Build history of the part. All positions in model axes, mm. Round coordinates to 2 decimals unless told otherwise and drop trailing zeros. Loops run counter-clockwise (first coordinate to the right, second up) from the corner with the lowest first, then second, coordinate; pieces in that order, holes last. Notation, with made-up numbers: (67, -7) -> (94, -7) arc R10 ccw to (94, 11) -> close; hole circle Ø9 at (-5.75, 30). An arc over 180 degrees is marked (long way). Put each result on its own line as item: value. Start each with the question number.
Item 1: Drill centre lines: probe 1 along X at (y, z) = (64, 114); probe 2 along Y at (x, z) = (22.5, 61.5); probe 3 along X at (y, z) = (94, 33.5). Where is each one in solid material? Low to high. Write a range as [from, to].
Item 2: Cut at B-B, the plane x = 59. List the corners of the cut face in (y, z), plus the area to 3 significant figures.
Item 3: Cut at A-A, the plane y = 12.5. List the corners of the cut face in (x, z).
Item 4: Cut at C-C, the plane z = 74.5. List the corners of the cut face in (x, y), plus the area to 3 significant figures.
Item 5: Cut at D-D, the plane y = 73.5. List the corners of the cut face in (x, z), plus the area to 3 significant figures.
```python
from build123d import *

# Parameters (mm, degrees)
F0_W      = 127
F0_H      = 127
F1_DEPTH  = 127
F4_DEPTH  = 127
F6_DEPTH  = 127
F8_DEPTH  = 127
F10_DEPTH = 127


with BuildPart() as f1:
    # F0 (on Top) → F1 (new body)
    with BuildSketch(Plane.XY):
        with Locations((63.5, 63.5)):
            Rectangle(F0_W, F0_H)
    extrude(amount=F1_DEPTH)

    # F3 (on face) → F4 (cut)
    with BuildSketch(Plane.XY.offset(127)):
        with BuildLine():
            ThreePointArc((95.688511, 95.936173), (62.707134, 109.585316), (29.707732, 95.979811))
            Line((29.707732, 95.979811), (62.676218, 62.838437))
            Line((62.676218, 62.838437), (95.688511, 95.936173))
        make_face()
        with BuildLine():
            Line((62.676218, 62.838437), (29.707732, 95.979811))
            ThreePointArc((29.707732, 95.979811), (15.929338, 62.869353), (29.663924, 29.7407))
            Line((29.663924, 29.7407), (62.676218, 62.838437))
        make_face()
        with BuildLine():
            Line((95.688511, 95.936173), (62.676218, 62.838437))
            Line((62.676218, 62.838437), (95.644703, 29.697063))
            ThreePointArc((95.644703, 29.697063), (105.841284, 44.892719), (109.423107, 62.838437))
            ThreePointArc((109.423107, 62.838437), (105.853143, 80.755602), (95.688511, 95.936173))
        make_face()
        with BuildLine():
            Line((95.644703, 29.697063), (62.676218, 62.838437))
            Line((62.676218, 62.838437), (29.663924, 29.7407))
            ThreePointArc((29.663924, 29.7407), (62.645301, 16.091557), (95.644703, 29.697063))
        make_face()
    extrude(amount=-F4_DEPTH, mode=Mode.SUBTRACT)

    # F5 (on face) → F6 (cut)
    with BuildSketch(Plane.YZ.offset(127)):
        with BuildLine():
            ThreePointArc((90.100624, 90.100624), (63.5, 101.118963), (36.899376, 90.100624))
            Line((36.899376, 90.100624), (63.5, 63.5))
            Line((63.5, 63.5), (90.100624, 90.100624))
        make_face()
        with BuildLine():
            Line((63.5, 63.5), (36.899376, 90.100624))
            ThreePointArc((36.899376, 90.100624), (25.881037, 63.5), (36.899376, 36.899376))
            Line((36.899376, 36.899376), (63.5, 63.5))
        make_face()
        with BuildLine():
            Line((90.100624, 90.100624), (63.5, 63.5))
            Line((63.5, 63.5), (90.100624, 36.899376))
            ThreePointArc((90.100624, 36.899376), (98.25539, 49.103846), (101.118963, 63.5))
            ThreePointArc((101.118963, 63.5), (98.25539, 77.896154), (90.100624, 90.100624))
        make_face()
        with BuildLine():
            Line((90.100624, 36.899376), (63.5, 63.5))
            Line((63.5, 63.5), (36.899376, 36.899376))
            ThreePointArc((36.899376, 36.899376), (63.5, 25.881037), (90.100624, 36.899376))
        make_face()
    extrude(amount=F6_DEPTH, mode=Mode.SUBTRACT)

    # F7 (on face) → F8 (cut)
    with BuildSketch(Plane.YZ.offset(127)):
        with BuildLine():
            ThreePointArc((92.47811, 92.47811), (63.5, 104.481236), (34.52189, 92.47811))
            Line((34.52189, 92.47811), (63.5, 63.5))
            Line((63.5, 63.5), (92.47811, 92.47811))
        make_face()
        with BuildLine():
            Line((63.5, 63.5), (34.52189, 92.47811))
            ThreePointArc((34.52189, 92.47811), (22.518764, 63.5), (34.52189, 34.52189))
            Line((34.52189, 34.52189), (63.5, 63.5))
        make_face()
        with BuildLine():
            Line((92.47811, 92.47811), (63.5, 63.5))
            Line((63.5, 63.5), (92.47811, 34.52189))
            ThreePointArc((92.47811, 34.52189), (101.361725, 47.81716), (104.481236, 63.5))
            ThreePointArc((104.481236, 63.5), (101.361725, 79.18284), (92.47811, 92.47811))
        make_face()
        with BuildLine():
            Line((92.47811, 34.52189), (63.5, 63.5))
            Line((63.5, 63.5), (34.52189, 34.52189))
            ThreePointArc((34.52189, 34.52189), (63.5, 22.518764), (92.47811, 34.52189))
        make_face()
    extrude(amount=F8_DEPTH, mode=Mode.SUBTRACT)

    # F9 (on face) → F10 (cut)
    with BuildSketch(Plane(origin=(0, 127, 0), x_dir=(-1, 0, 0), z_dir=(0, 1, 0))):
        with BuildLine():
            ThreePointArc((-90.440768, 90.440768), (-101.6, 63.5), (-90.440768, 36.559232))
            Line((-90.440768, 36.559232), (-63.5, 63.5))
            Line((-63.5, 63.5), (-90.440768, 90.440768))
        make_face()
        with BuildLine():
            Line((-63.5, 63.5), (-90.440768, 36.559232))
            ThreePointArc((-90.440768, 36.559232), (-63.5, 25.4), (-36.559232, 36.559232))
            Line((-36.559232, 36.559232), (-63.5, 63.5))
        make_face()
        with BuildLine():
            Line((-90.440768, 90.440768), (-63.5, 63.5))
            Line((-63.5, 63.5), (-36.559232, 90.440768))
            ThreePointArc((-36.559232, 90.440768), (-63.5, 101.6), (-90.440768, 90.440768))
        make_face()
        with BuildLine():
            Line((-36.559232, 90.440768), (-63.5, 63.5))
            Line((-63.5, 63.5), (-36.559232, 36.559232))
            ThreePointArc((-36.559232, 36.559232), (-28.30019, 48.919761), (-25.4, 63.5))
            ThreePointArc((-25.4, 63.5), (-28.30019, 78.080239), (-36.559232, 90.440768))
        make_face()
    extrude(amount=-F10_DEPTH, mode=Mode.SUBTRACT)


solid = f1.part
```
Reply:
1. probe 1: x = [0, 15.94], [109.41, 127]
1. probe 2: y = [0, 38.94], [86.74, 127]
1. probe 3: x = [0, 27.83], [97.52, 127]
2. outline: (0, 0) -> (16.24, 0) -> (16.24, 25.67) -> (0, 25.67) -> close; (0, 101.33) -> (16.24, 101.33) -> (16.24, 127) -> (0, 127) -> close; (109.44, 0) -> (127, 0) -> (127, 25.67) -> (109.44, 25.67) -> close; (109.44, 101.33) -> (127, 101.33) -> (127, 127) -> (109.44, 127) -> close
2. area: 1,730 mm^2
3. outline: (0, 0) -> (127, 0) -> (127, 127) -> (0, 127) -> close; hole (36.56, 36.56) arc R38.1 ccw to (90.44, 36.56) arc R38.1 ccw to (90.44, 90.44) arc R38.1 ccw to (36.56, 90.44) arc R38.1 ccw to start
4. outline: (0, 0) -> (27.02, 0) -> (27.02, 32.6) arc R46.75 cw to (27.02, 93.07) -> (27.02, 127) -> (0, 127) -> close; (99.98, 0) -> (127, 0) -> (127, 127) -> (99.98, 127) -> (99.98, 91.01) arc R46.75 cw to (109.42, 62.84) arc R46.75 cw to (99.98, 34.66) -> close
4. area: 6,040 mm^2
5. outline: (0, 0) -> (17.16, 0) -> (17.16, 127) -> (0, 127) -> close; (108.19, 0) -> (127, 0) -> (127, 127) -> (108.19, 127) -> close
5. area: 4,570 mm^2
